Part model, mm, in its own coordinate system. Face numbers are marked on the shaded views. A direction names the side the tool comes from. Coordinates: 2 decimals unless noted, no trailing zeros. Order: outer loops, then holes, each group sorted by start corner. A loop starts at its lowest first (then second) coordinate and runs counter-clockwise, first axis right, second up.
1) Wall check: L1, parallel to X at y = 33, z = 0; L2, parallel to X at y = 19.5, z = 61; L3, parallel to X at y = 54, z = 5. Give the ranges that are in metal, low to high.
2) Cut at C-C (x = 0). List the corners of the cut face in (y, z).
3) Cut at B-B (z = 0). List the corners of the cut face in (x, y).
4) Cut at D-D (y = 69.5). List the corners of the cut face in (x, z).
5) Pin check, flat tips, straight feed: pin 1 Ø10 at (y, z) = (34.5, 45.5) entering from -X; pin 2 Ø7.5 at (x, y) = (-49, 37.5) entering from -Z; pin 3 Ø2 at (y, z) = (46.5, 14) entering from -X. Stop position of each tip, or through.
6) Mould opens along X. For the marked faces 6, 7 and 8 say: +X half, -X half, draft (parallel to the pull), parting line (faces both ways), or undercut.
7) Tool access for the marked faces 1, 2, 3, 4 and 5: list every direction of +Z, -Z, +X, -X, +Y, -Y with a clear straight run to the whole face (end or side of a thin tool).
8) Cut at A-A (y = 37.5). List the corners of the cut face in (x, z) (3 decimals).
```python
from build123d import *

# Parameters (mm, degrees)
SKETCH1_R                      = 35
SKETCH1_R_2                    = 20
BOSS_EXTRUDE2_DEPTH            = 75
CUT_EXTRUDE1_REACH             = 142.496
SKETCH2_R                      = 8.5
CUT_EXTRUDE1_DIRECTION_2_DEPTH = 141.496441236
FILLET1_R                      = 30


with BuildPart() as part:
    # Sketch1 → Boss-Extrude2 (new body)
    # profile 1 of 4: a face of its own
    with BuildSketch(Plane(origin=(0, 0, 0), x_dir=(1, 0, 0), z_dir=(0, 1, 0))):
        Circle(SKETCH1_R)
        with Locations(Location((0, 0, 0), (0, 0, 270))):
            Circle(SKETCH1_R_2, mode=Mode.SUBTRACT)
    # profile 2 of 4: a face of its own
    with BuildSketch(Plane(origin=(0, 0, 0), x_dir=(1, 0, 0), z_dir=(0, 1, 0))):
        with BuildLine():
            ThreePointArc((-55, 17), (-72, 0), (-55, -17))
            Line((-55, -17), (-30.594117082, -17))
            ThreePointArc((-30.594117082, -17), (-32.736987087, -12.381020816), (-34.186985828, -7.5))
            Line((-34.186985828, -7.5), (-55, -7.5))
            ThreePointArc((-55, -7.5), (-62.5, 0), (-55, 7.5))
            Line((-55, 7.5), (-34.186985828, 7.5))
            ThreePointArc((-34.186985828, 7.5), (-32.736987087, 12.381020816), (-30.594117082, 17))
            Line((-30.594117082, 17), (-55, 17))
        make_face()
    # profile 3 of 4: a face of its own
    with BuildSketch(Plane(origin=(0, 0, 0), x_dir=(1, 0, 0), z_dir=(0, 1, 0))):
        with BuildLine():
            ThreePointArc((-7.5, -34.186985828), (-15.446901808, -31.406897722), (-22.5, -26.809513237))
            Line((-22.5, -26.809513237), (-22.5, -72))
            Line((-22.5, -72), (-7.5, -72))
            Line((-7.5, -72), (-7.5, -34.186985828))
        make_face()
    # profile 4 of 4: a face of its own
    with BuildSketch(Plane(origin=(0, 0, 0), x_dir=(1, 0, 0), z_dir=(0, 1, 0))):
        with BuildLine():
            ThreePointArc((22.5, -26.809513237), (15.446901808, -31.406897722), (7.5, -34.186985828))
            Line((7.5, -34.186985828), (7.5, -72))
            Line((7.5, -72), (22.5, -72))
            Line((22.5, -72), (22.5, -26.809513237))
        make_face()
    extrude(amount=BOSS_EXTRUDE2_DEPTH)

    # Cut-Extrude1: up to this face of the body (flat: up to its plane)
    cut_extrude1_end = Plane(part.part.faces().sort_by_distance((-22.5, 37.5, 49.404756618))[0])
    # Sketch2 → Cut-Extrude1 (cut, up to the picked face)
    with BuildSketch(Plane(origin=(22.5, 0, 0), x_dir=(0, 0, -1), z_dir=(1, 0, 0)), mode=Mode.PRIVATE) as cut_extrude1_sk1:
        with Locations((-49.405, 37.5)):
            Circle(SKETCH2_R)
    cut_extrude1_tool1 = split(extrude(cut_extrude1_sk1.sketch, amount=-CUT_EXTRUDE1_REACH, mode=Mode.PRIVATE), bisect_by=cut_extrude1_end, keep=Keep.BOTH, mode=Mode.PRIVATE)
    add(cut_extrude1_tool1.solids().sort_by(Axis((22.5, 37.5, 49.405), (-1, 0, 0)))[0], mode=Mode.SUBTRACT)

    # Sketch2 → Cut-Extrude1 direction 2 (cut)
    with BuildSketch(Plane(origin=(22.5, 0, 0), x_dir=(0, 0, -1), z_dir=(1, 0, 0))):
        with Locations((-49.405, 37.5)):
            Circle(SKETCH2_R)
    extrude(amount=CUT_EXTRUDE1_DIRECTION_2_DEPTH, mode=Mode.SUBTRACT)

    # Fillet1
    fillet1_edges = [part.edges().sort_by_distance(p)[0] for p in [
        (-15, 0, 72),
        (15, 0, 72),
        (15, 75, 72),
        (-15, 75, 72),
    ]]
    fillet(fillet1_edges, radius=FILLET1_R)


solid = part.part
```
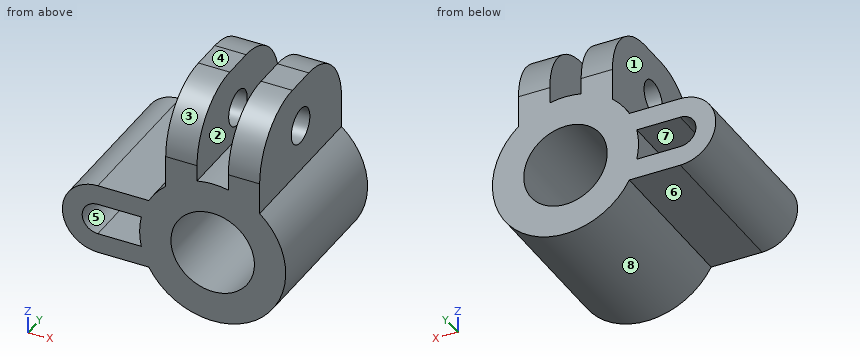
Geometry check:
1. L1: x = -72 to -62.5, -35 to -20, 20 to 35
1. L2: x = -22.5 to -7.5, 7.5 to 22.5
1. L3: x = -71.25 to -60.59, -34.64 to -19.36, 19.36 to 34.64
2. outline: (0, -35) - (75, -35) - (75, -20) - (0, -20) - close; (0, 20) - (75, 20) - (75, 35) - (0, 35) - close
3. outline: (-72, 0) - (-62.5, 0) - (-62.5, 75) - (-72, 75) - close; (-35, 0) - (-20, 0) - (-20, 75) - (-35, 75) - close; (20, 0) - (35, 0) - (35, 75) - (20, 75) - close
4. outline: (-55, -17) - (-30.59, -17) arc R35 ccw (long way) to (22.5, 26.81) - (22.5, 59.31) - (7.5, 59.31) - (7.5, 34.19) arc R35 ccw to (-7.5, 34.19) - (-7.5, 59.31) - (-22.5, 59.31) - (-22.5, 26.81) arc R35 ccw to (-30.59, 17) - (-55, 17) arc R17 ccw to start; hole (-55, -7.5) - (-34.19, -7.5) arc R35 cw to (-34.19, 7.5) - (-55, 7.5) arc R7.5 ccw to start; hole circle Ø40 at (0, 0)
5. pin 1: stops at x = -22.5
5. pin 2: stops at z = -17
5. pin 3: stops at x = -65.95
6. face 6: draft
6. face 7: undercut
6. face 8: parting line
7. face 1: +Z, -X, +Y, -Y
7. face 2: +Z, +Y, -Y
7. face 3: +Z, +X, -X, -Y
7. face 4: +Z, +X, -X, +Y, -Y
7. face 5: +Y, -Y
8. outline: (-55, -17) - (-30.594, -17) arc R35 ccw (long way) to (22.5, 26.81) - (22.5, 40.905) - (7.5, 40.905) - (7.5, 34.187) arc R35 ccw to (-7.5, 34.187) - (-7.5, 40.905) - (-22.5, 40.905) - (-22.5, 26.81) arc R35 ccw to (-30.594, 17) - (-55, 17) arc R17 ccw to start; (-22.5, 57.905) - (-7.5, 57.905) - (-7.5, 72) - (-22.5, 72) - close; (7.5, 57.905) - (22.5, 57.905) - (22.5, 72) - (7.5, 72) - close; hole (-55, -7.5) - (-34.187, -7.5) arc R35 cw to (-34.187, 7.5) - (-55, 7.5) arc R7.5 ccw to start; hole circle Ø40 at (0, 0)
